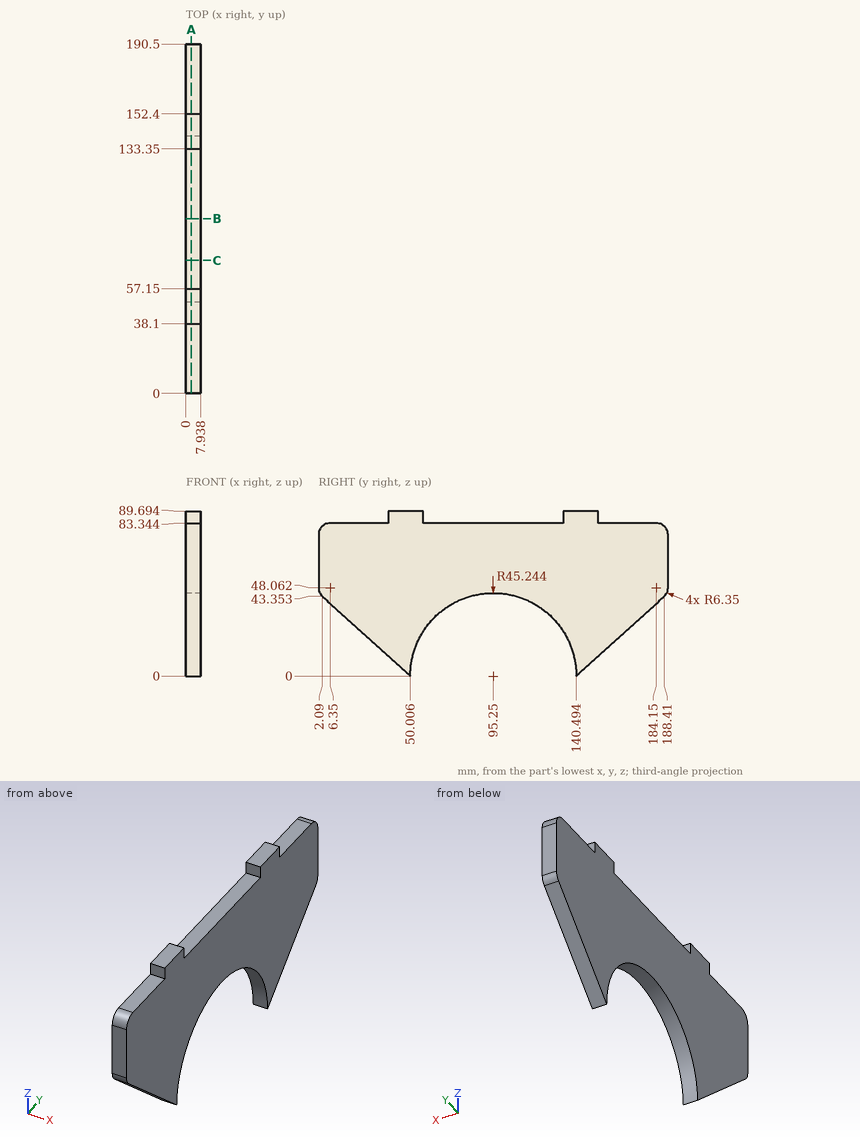
The drawing under review shows one solid part. Ordinate dimensions are in mm from its lowest x, y, z. Coordinates: 2 decimals unless noted, no trailing zeros. Loops run counter-clockwise (first coordinate to the right, second up) from the corner with the lowest first, then second, coordinate; pieces in that order, holes last. Notation, with made-up numbers: M -12.75,5 L 24.25,5 A28 cw 24.25,27 Z; hole C 5,71.25 d9. An arc over 180 degrees is marked long. Use one line per item in the form item = value.
(1) For line 1 along Y through (x, z) = (3.5, 37) (1 decimal); line 2 along Y through (x, z) = (1.5, 16) (1 decimal); line 3 along Y through (x, z) = (3.25, 47.5) (1 decimal), list the stretches that pass through material, from the lowest coordinate up. Write a range as from..to.
Return value:
line_1 = 9.1..69.2, 121.3..181.4
line_2 = 32.3..52.9, 137.6..158.2
line_3 = 0..190.5
(2) Consider section B-B (y = 95.25). Write out the cut boundary in (x, z).
Return value:
outline = M 0,45.24 L 7.94,45.24 L 7.94,83.34 L 0,83.34 Z
(3) Consider section A-A (x = 3). Write out the cut boundary in (y, z), and give its area (3 significant figures).
Return value:
outline = M 0,48.06 A6.35 ccw 2.09,43.35 L 50.01,0 A45.24 cw 140.49,0 L 188.41,43.35 A6.35 ccw 190.5,48.06 L 190.5,76.99 A6.35 ccw 184.15,83.34 L 152.4,83.34 L 152.4,89.69 L 133.35,89.69 L 133.35,83.34 L 57.15,83.34 L 57.15,89.69 L 38.1,89.69 L 38.1,83.34 L 6.35,83.34 A6.35 ccw 0,76.99 Z
area = 10,600 mm2
(4) Consider section C-C (y = 72.5). Write out the cut boundary in (x, z).
Return value:
outline = M 0,39.11 L 7.94,39.11 L 7.94,83.34 L 0,83.34 Z
(5) Clearance check with flat-ended pins moving along their axes: P1, Ø4, axis at x = 3, y = 109, coming from the +Z side; P2, Ø3, axis at x = 5.5, z = 86.5, coming from the +Y side; P3, Ø1, axis at x = 6, z = 25.5, coming from the +Y side. State where each tip first meets the part, or that it passes through.
Return value:
P1 = 83.34
P2 = 152.4
P3 = 169.23
